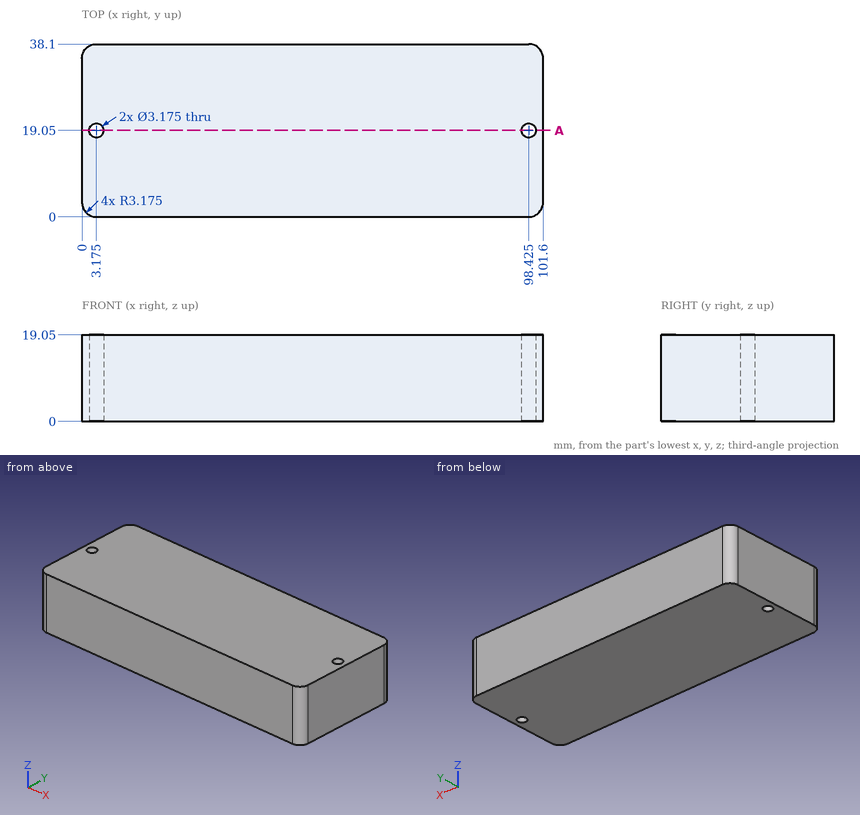
The figure shows three views and two pictorial views of one solid part (mm, origin at its lowest corner). Answer the questions. Coordinates: 2 decimals unless noted, no trailing zeros. Loops run counter-clockwise (first coordinate to the right, second up) from the corner with the lowest first, then second, coordinate; pieces in that order, holes last. Notation, with made-up numbers: (14.25, -3) - (36.25, -3) arc R23 cw to (36.25, 9) - close; hole circle Ø3 at (-27, 57.5). An arc over 180 degrees is marked (long way). Answer in a Markdown table with one row per item.
Q1. Find section A-A on y = 19.05. Write down the section's boundary in (x, z), plus the area to 3 significant figures.
Here are the results:
| item | result |
|---|---|
| outline | (0, 0) - (1.59, 0) - (1.59, 19.05) - (0, 19.05) - close; (4.76, 0) - (96.84, 0) - (96.84, 19.05) - (4.76, 19.05) - close; (100.01, 0) - (101.6, 0) - (101.6, 19.05) - (100.01, 19.05) - close |
| area | 1,810 mm^2 |
Q2. Given P1, Ø3, axis at x = 98.425, y = 19.05, coming from the -Z side, flat-ended and moving along its own axis, determine where the tip first touches the part or whether it passes through.
Here are the results:
| item | result |
|---|---|
| P1 | passes through |
Q3. Straight lines are drawn through the part: line 1 along X through (y, z) = (20, 1); line 2 along X through (y, z) = (2, 5); line 3 along X through (y, z) = (35.5, 15). For each, find the intervals that lie inside material, in ascending order. Write a range as [from, to].
Here are the results:
| item | result |
|---|---|
| line 1 | x = [0, 1.9], [4.45, 97.15], [99.7, 101.6] |
| line 2 | x = [0.23, 101.37] |
| line 3 | x = [0.05, 101.55] |
